Design review of the part built by this model. Coordinates are the model's own, in mm. A direction names the side the tool comes from. Round coordinates to 2 decimals unless told otherwise and drop trailing zeros. Order: outer loops, then holes, each group sorted by start corner. A loop starts at its lowest first (then second) coordinate and runs counter-clockwise, first axis right, second up. Notation, with made-up numbers: (24.5, 50.25) - (43.5, 50.25) arc R21 cw to (43.5, 87.25) - close; hole circle Ø11 at (20, 40). An arc over 180 degrees is marked (long way). Write item = value, one per line.
from build123d import *

# Parameters (mm, degrees)
SKETCH1_R           = 10
BOSS_EXTRUDE1_DEPTH = 4
SKETCH2_R           = 5.25
BOSS_EXTRUDE2_DEPTH = 4
SKETCH3_R           = 1.35
CUT_EXTRUDE1_DEPTH  = 15.696938457
SKETCH4_R           = 4
CUT_EXTRUDE2_DEPTH  = 17.248076809


with BuildPart() as part:
    # Sketch1 → Boss-Extrude1 (new body)
    with BuildSketch(Plane(origin=(0, 0, 0), x_dir=(1, 0, 0), z_dir=(0, 1, 0))):
        with Locations(Location((0, 0, 0), (0, 0, 270))):
            Circle(SKETCH1_R)
    extrude(amount=BOSS_EXTRUDE1_DEPTH)

    # Sketch2 → Boss-Extrude2 (add)
    with BuildSketch(Plane(origin=(0, 4, 0), x_dir=(1, 0, 0), z_dir=(0, 1, 0))):
        with Locations(Location((0, 0, 0), (0, 0, 270))):
            Circle(SKETCH2_R)
    extrude(amount=BOSS_EXTRUDE2_DEPTH)

    # Sketch3 → Cut-Extrude1 (cut, through all)
    with BuildSketch(Plane(origin=(0, 4, 0), x_dir=(1, 0, 0), z_dir=(0, 1, 0))):
        with Locations(Location((0, 7.5, 0), (0, 0, 270))):
            Circle(SKETCH3_R)
        with Locations(Location((7.5, 0, 0), (0, 0, 270))):
            Circle(SKETCH3_R)
        with Locations(Location((0, -7.5, 0), (0, 0, 90))):
            Circle(SKETCH3_R)
        with Locations(Location((-7.5, 0, 0), (0, 0, 90))):
            Circle(SKETCH3_R)
    extrude(amount=-CUT_EXTRUDE1_DEPTH, mode=Mode.SUBTRACT)

    # Sketch4 → Cut-Extrude2 (cut, through all)
    with BuildSketch(Plane(origin=(0, 8, 0), x_dir=(-1, 0, 0), z_dir=(0, 1, 0))):
        with Locations(Location((0, 0, 0), (0, 0, 90))):
            Circle(SKETCH4_R)
    extrude(amount=-CUT_EXTRUDE2_DEPTH, mode=Mode.SUBTRACT)


solid = part.part
Item 1: Insertion check: P1, Ø1, axis at x = -2.5, y = 3, coming from the -Z side; P2, Ø2, axis at y = 4.5, z = 4.5, coming from the +X side; P3, Ø1.5, axis at x = 1, y = 4.5, coming from the +Z side. Each pin has a flat end and moves straight along its axis. Give the tip position at first contact, or say it passes through.
Data:
P1 = -9.8
P2 = 9.32
P3 = 9.99
Item 2: For line 1 along X through (y, z) = (2.3, 0); line 2 along Z through (x, y) = (-0.5, 5); line 3 along X through (y, z) = (1.45, -7.5), list the stretches that pass through material, from the lowest coordinate up. Write a range as [from, to].
Data:
line_1 = [-10, -8.85], [-6.15, -4], [4, 6.15], [8.85, 10]
line_2 = [-5.23, -3.97], [3.97, 5.23]
line_3 = [-6.61, -1.35], [1.35, 6.61]
Item 3: The part is to be moulded in two halves that separate along Z. For faces 3 (the face through (1.6, 6, 5)), 4 (the face through (-2, 8, -4)), 5 (the face through (-3.905, 4.056, -0.867)), say which applies: +Z half, -Z half, draft (parallel to the pull), parting line (faces both ways), or undercut.
Data:
face_3 = parting line
face_4 = draft
face_5 = undercut
Item 4: Take a section at B-B, the plane x = -7.5. State the section outline as (y, z) points.
Data:
outline = (0, -6.61) - (4, -6.61) - (4, -1.35) - (0, -1.35) - close; (0, 1.35) - (4, 1.35) - (4, 6.61) - (0, 6.61) - close
Item 5: For faces 1 (the face through (-4, 4, 4)), 2 (the face through (0.1, 0, 4.3)), list the 3-axis set-ups (+Z, -Z, +X, -X, +Y, -Y) from which the entire face can be reached by the end or side of a thin tool; tool diameter is ignored.
Data:
face_1 = +Y
face_2 = +Z, -Z, +X, -X, -Y
Item 6: Take a section at D-D, the plane y = 2.75. State the section outline as (x, z) points, and give its area (3 significant figures).
Data:
outline = circle Ø20 at (0, 0); hole circle Ø2.7 at (-7.5, 0); hole circle Ø8 at (0, 0); hole circle Ø2.7 at (0, -7.5); hole circle Ø2.7 at (0, 7.5); hole circle Ø2.7 at (7.5, 0)
area = 241 mm2
Item 7: Take a section at A-A, the plane z = 0. State the section outline as (x, y) points.
Data:
outline = (-10, 0) - (-8.85, 0) - (-8.85, 4) - (-10, 4) - close; (-6.15, 0) - (-4, 0) - (-4, 8) - (-5.25, 8) - (-5.25, 4) - (-6.15, 4) - close; (4, 0) - (6.15, 0) - (6.15, 4) - (5.25, 4) - (5.25, 8) - (4, 8) - close; (8.85, 0) - (10, 0) - (10, 4) - (8.85, 4) - close
Item 8: Take a section at C-C, the plane z = 6.75. State the section outline as (x, y) points, and give its area (3 significant figures).
Data:
outline = (-7.38, 0) - (-1.12, 0) - (-1.12, 4) - (-7.38, 4) - close; (1.12, 0) - (7.38, 0) - (7.38, 4) - (1.12, 4) - close
area = 50.0 mm2
